from build123d import *

# Parameters (mm, degrees)
SKETCH_1_W          = 129.5
SKETCH_1_H          = 204.5
EXTRUDE_1_DEPTH     = 6.75
SKETCH_2_W          = 129.5
SKETCH_2_H          = 8
CUT_EXTRUDE_1_DEPTH = 4
SKETCH_3_R          = 2.35
EXTRUDE_2_DEPTH     = 8.5
SKETCH_4_W          = 120
SKETCH_4_H          = 175
CUT_EXTRUDE_3_DEPTH = 5
SKETCH_5_W          = 9.7
SKETCH_5_H          = 215
EXTRUDE_3_DEPTH     = 2.75
SKETCH_6_W          = 50
SKETCH_6_H          = 15
EXTRUDE_4_DEPTH     = 4
SKETCH_7_W          = 46
SKETCH_7_H          = 2
CUT_EXTRUDE_4_DEPTH = 13
SKETCH_8_W          = 15
SKETCH_8_H          = 15
CUT_EXTRUDE_5_DEPTH = 4
SKETCH_9_W          = 76
SKETCH_9_H          = 29
EXTRUDE_5_DEPTH     = 20
SKETCH_10_W         = 9.7
SKETCH_10_H         = 175
CUT_EXTRUDE_6_DEPTH = 1
SKETCH_11_W         = 71
SKETCH_11_H         = 25.5
CUT_EXTRUDE_8_DEPTH = 20.2


with BuildPart() as part:
    # 草图1 → 凸台-拉伸1 (new body)
    with BuildSketch(Plane(origin=(0, 0, 0), x_dir=(1, 0, 0), z_dir=(0, 1, 0))):
        Rectangle(SKETCH_1_W, SKETCH_1_H)
    extrude(amount=EXTRUDE_1_DEPTH)

    # 草图2 → 切除-拉伸1 (cut)
    with BuildSketch(Plane.XZ):
        with Locations((0, 98.25)):
            Rectangle(SKETCH_2_W, SKETCH_2_H)
        with Locations((0, -98.25)):
            Rectangle(SKETCH_2_W, SKETCH_2_H)
    extrude(amount=-CUT_EXTRUDE_1_DEPTH, mode=Mode.SUBTRACT)

    # 草图3 → 凸台-拉伸2 (add)
    with BuildSketch(Plane.XZ.offset(-4)):
        with Locations(Location((-61, 98.5, 0), (0, 0, 270))):
            Circle(SKETCH_3_R)
        with Locations(Location((61, 98.5, 0), (0, 0, 270))):
            Circle(SKETCH_3_R)
        with Locations(Location((61, -98.5, 0), (0, 0, 90))):
            Circle(SKETCH_3_R)
        with Locations(Location((-61, -98.5, 0), (0, 0, 90))):
            Circle(SKETCH_3_R)
    extrude(amount=EXTRUDE_2_DEPTH)

    # 草图4 → 切除-拉伸3 (cut)
    with BuildSketch(Plane.XZ):
        with Locations((4.75, 0)):
            Rectangle(SKETCH_4_W, SKETCH_4_H)
    extrude(amount=-CUT_EXTRUDE_3_DEPTH, mode=Mode.SUBTRACT)

    # 草图5 → 凸台-拉伸3 (add)
    with BuildSketch(Plane(origin=(0, 6.75, 0), x_dir=(1, 0, 0), z_dir=(0, 1, 0))):
        Rectangle(SKETCH_5_W, SKETCH_5_H)
    extrude(amount=-EXTRUDE_3_DEPTH)

    # 草图6 → 凸台-拉伸4 (add)
    with BuildSketch(Plane(origin=(0, 6.75, 0), x_dir=(1, 0, 0), z_dir=(0, 1, 0))):
        Rectangle(SKETCH_6_W, SKETCH_6_H)
    extrude(amount=EXTRUDE_4_DEPTH)

    # 草图7 → 切除-拉伸4 (cut)
    with BuildSketch(Plane.XY.offset(7.5)):
        with Locations((0, 7.75)):
            Rectangle(SKETCH_7_W, SKETCH_7_H)
    extrude(amount=-CUT_EXTRUDE_4_DEPTH, mode=Mode.SUBTRACT)

    # 草图8 → 切除-拉伸5 (cut)
    with BuildSketch(Plane(origin=(0, 10.75, 0), x_dir=(1, 0, 0), z_dir=(0, 1, 0))):
        Rectangle(SKETCH_8_W, SKETCH_8_H)
    extrude(amount=-CUT_EXTRUDE_5_DEPTH, mode=Mode.SUBTRACT)

    # 草图9 → 凸台-拉伸5 (add)
    with BuildSketch(Plane(origin=(0, 6.75, 0), x_dir=(1, 0, 0), z_dir=(0, 1, 0))):
        with Locations((0, 22)):
            Rectangle(SKETCH_9_W, SKETCH_9_H)
    extrude(amount=EXTRUDE_5_DEPTH)

    # 草图10 → 切除-拉伸6 (cut)
    with BuildSketch(Plane.XZ.offset(-4)):
        Rectangle(SKETCH_10_W, SKETCH_10_H)
    extrude(amount=-CUT_EXTRUDE_6_DEPTH, mode=Mode.SUBTRACT)

    # 草图11 → 切除-拉伸8 (cut)
    with BuildSketch(Plane.XZ.offset(-5)):
        with Locations((0, -22)):
            Rectangle(SKETCH_11_W, SKETCH_11_H)
    extrude(amount=-CUT_EXTRUDE_8_DEPTH, mode=Mode.SUBTRACT)


solid = part.part
Can you work these out from the model? Positions are in its coordinate system, mm. A direction names the side the tool comes from. Round coordinates to 2 decimals unless told otherwise and drop trailing zeros. Order: outer loops, then holes, each group sorted by start corner. A loop starts at its lowest first (then second) coordinate and runs counter-clockwise, first axis right, second up. Notation, with made-up numbers: M 61,10 L 73,10 A21 ccw 73,24 Z; hole C 67.5,-18.75 d9. An arc over 180 degrees is marked long. Use a Markdown table: item, result.
1) Imagine slicing it at A-A (y = 20.5). List the corners of the cut face in (x, z) for me, then the cut area to 4 significant figures.
Geometry says:
| item | result |
|---|---|
| outline | M -38,-36.5 L 38,-36.5 L 38,-7.5 L -38,-7.5 Z; hole M -35.5,-34.75 L 35.5,-34.75 L 35.5,-9.25 L -35.5,-9.25 Z |
| area | 393.5 mm² |
2) If I drill on line 1 along X through (y, z) = (17, -28); line 2 along Z through (x, y) = (15.5, 6); line 3 along Z through (x, y) = (-18.5, 18), over which ranges is the centre line in solid material (lowest first)?
Geometry says:
| item | result |
|---|---|
| line 1 | x = -38 to -35.5, 35.5 to 38 |
| line 2 | z = -102.25 to -34.75, -9.25 to 102.25 |
| line 3 | z = -36.5 to -34.75, -9.25 to -7.5 |
3) Imagine slicing it at C-C (z = 98.5). List the corners of the cut face in (x, y) for me.
Geometry says:
| item | result |
|---|---|
| outline | M -64.75,4 L -63.35,4 L -63.35,-4.5 L -58.65,-4.5 L -58.65,4 L 58.65,4 L 58.65,-4.5 L 63.35,-4.5 L 63.35,4 L 64.75,4 L 64.75,6.75 L -64.75,6.75 Z |
4) I'm going to push flat-ended pins straight in: P1, Ø2, axis at x = 4.5, y = 22, coming from the -Z side; P2, Ø1.5, axis at x = 6.5, y = 1, coming from the +Z side; P3, Ø1.2, axis at x = -15.5, y = 8, coming from the +Z side. Where does each tip first touch, or does it pass through?
Geometry says:
| item | result |
|---|---|
| P1 | stops at z = -36.5 |
| P2 | stops at z = 94.25 |
| P3 | stops at z = -5.5 |
5) Imagine slicing it at B-B (x = -1). List the corners of the cut face in (y, z) for me.
Geometry says:
| item | result |
|---|---|
| outline | M 0,-94.25 L 4,-94.25 L 4,-107.5 L 6.75,-107.5 L 6.75,-36.5 L 26.75,-36.5 L 26.75,-7.5 L 6.75,-7.5 L 6.75,107.5 L 4,107.5 L 4,94.25 L 0,94.25 L 0,87.5 L 5,87.5 L 5,-9.25 L 25.2,-9.25 L 25.2,-34.75 L 5,-34.75 L 5,-87.5 L 0,-87.5 Z |
6) On a 3-axis mill with a long thin cutter (end or side, diameter ignored), from which of +Z, -Z, +X, -X, +Y, -Y can I reach the whole of each face in a straight line? I mean faces 1 (the face through (38, 17, -22)), 2 (the face through (-58, 0, 0)), 3 (the face through (0, 15, -9.25)), 4 (the face through (-15, 8.75, 1)), 5 (the face through (-1, 17, -36.5)). Say none if no direction works.
Geometry says:
| item | result |
|---|---|
| face 1 | +Z, -Z, +X, +Y |
| face 2 | +X, -X, -Y |
| face 3 | -Y |
| face 4 | +Z |
| face 5 | -Z, +X, -X, +Y |
7) Imagine slicing it at D-D (x = 61). List the corners of the cut face in (y, z) for me, then the cut area to 3 significant figures.
Geometry says:
| item | result |
|---|---|
| outline | M -4.5,-100.85 L 4,-100.85 L 4,-102.25 L 6.75,-102.25 L 6.75,102.25 L 4,102.25 L 4,100.85 L -4.5,100.85 L -4.5,96.15 L 4,96.15 L 4,94.25 L 0,94.25 L 0,87.5 L 5,87.5 L 5,-87.5 L 0,-87.5 L 0,-94.25 L 4,-94.25 L 4,-96.15 L -4.5,-96.15 Z |
| area | 521 mm² |
8) If we mould it in two halves opening along X, with no side actions, what happens to faces 6 (the face through (-38, 17, -22)), 7 (the face through (4, 2, 87.5)), 8 (the face through (7.5, 10, 0))? For each: +X half, -X half, draft (parallel to the pull), parting line (faces both ways), or undercut.
Geometry says:
| item | result |
|---|---|
| face 6 | -X half |
| face 7 | draft |
| face 8 | undercut |
